from build123d import *

# Parameters (mm, degrees)
F0_W     = 76.2
F0_H     = 76.2
F0_W_2   = 63.5
F0_H_2   = 63.5
F1_DEPTH = 584.2
F3_D     = 12.7


# Not quite as in the source:
# - a length typed as a fraction of an inch, garbled in the dataset ("3 / 203.2 mm" for 3/8 in), is restored


with BuildPart() as f1:
    # F0 (on Top) → F1 (new body)
    with BuildSketch(Plane.XY):
        Rectangle(F0_W, F0_H)
        Rectangle(F0_W_2, F0_H_2, mode=Mode.SUBTRACT)
    extrude(amount=F1_DEPTH)

    # F3 (through all)
    with Locations(Plane.XZ.offset(38.1)):
        with Locations((0, 533.4)):
            Hole(F3_D / 2)


solid = f1.part
Can you work these out from the model? Positions are in its coordinate system, mm. A direction names the side the tool comes from. Round coordinates to 2 decimals unless told otherwise and drop trailing zeros. Write each loop counter-clockwise with the first axis right and the second up, starting at its lowest first coordinate (ties: lowest second). Pieces come first, ordered by that corner, then holes. Notation, with made-up numbers: (-6, 82.25) -> (16, 82.25) arc R13 ccw to (16, 106.25) -> close; hole circle Ø3 at (-17.5, 72.5). An arc over 180 degrees is marked (long way). Use one line per item in the form item = value. Start each with the question number.
Q1. Imagine slicing it at C-C (z = 533.4). Please give me the cut outline in (x, y), then the cut area to 3 significant figures.
Q2. Which directions (+Z, -Z, +X, -X, +Y, -Y) give clear straight access to the entire face, cutting with the end or side of a thin tool? Please do faces 1 (the face through (-1, 38.1, 288)), 2 (the face through (-31.75, 0, 288)).
Q3. Imagine slicing it at D-D (x = 0). Please give me the cut outline in (y, z), then the cut area to 3 significant figures.
Q4. If I drill on probe 1 along Z at (x, y) = (0, -34); probe 2 along Y at (x, z) = (-21, 257.5), over which ranges is the centre line in solid material (lowest first)? Write a range as [from, to].
Q5. We'd pull the mould along Z, two halves only. Please class faces 3 (the face through (0.8, -34.9, 539.7)), 4 (the face through (31.75, 0, 288)), 5 (the face through (-34, 1, 584.2)), 6 (the face through (0.8, 35, 539.7)): +Z half, -Z half, draft (parallel to the pull), parting line (faces both ways), or undercut.
Q6. Imagine slicing it at A-A (x = -26.5). Please give me the cut outline in (y, z).
Q7. I'm going to push a flat-ended pin straight in: P1, Ø16.5, axis at x = 0, z = 533.4, coming from the +Y side. Where does the tip first touch, or does it pass through?
Worked out:
q1.outline = (-38.1, -38.1) -> (-6.35, -38.1) -> (-6.35, -31.75) -> (-31.75, -31.75) -> (-31.75, 31.75) -> (-6.35, 31.75) -> (-6.35, 38.1) -> (-38.1, 38.1) -> close; (6.35, -38.1) -> (38.1, -38.1) -> (38.1, 38.1) -> (6.35, 38.1) -> (6.35, 31.75) -> (31.75, 31.75) -> (31.75, -31.75) -> (6.35, -31.75) -> close
q1.area = 1,610 mm^2
q2.face_1 = +Z, -Z, +X, -X, +Y
q2.face_2 = +Z, -Z
q3.outline = (-38.1, 0) -> (-31.75, 0) -> (-31.75, 527.05) -> (-38.1, 527.05) -> close; (-38.1, 539.75) -> (-31.75, 539.75) -> (-31.75, 584.2) -> (-38.1, 584.2) -> close; (31.75, 0) -> (38.1, 0) -> (38.1, 527.05) -> (31.75, 527.05) -> close; (31.75, 539.75) -> (38.1, 539.75) -> (38.1, 584.2) -> (31.75, 584.2) -> close
q3.area = 7,260 mm^2
q4.probe_1 = [0, 527.05], [539.75, 584.2]
q4.probe_2 = [-38.1, -31.75], [31.75, 38.1]
q5.face_3 = undercut
q5.face_4 = draft
q5.face_5 = +Z half
q5.face_6 = undercut
q6.outline = (-38.1, 0) -> (-31.75, 0) -> (-31.75, 584.2) -> (-38.1, 584.2) -> close; (31.75, 0) -> (38.1, 0) -> (38.1, 584.2) -> (31.75, 584.2) -> close
q7.P1 = 38.1
